Geometry: final body of the model. Coordinates: model frame, mm. Round coordinates to 2 decimals unless told otherwise and drop trailing zeros. Loops run counter-clockwise (first coordinate to the right, second up) from the corner with the lowest first, then second, coordinate; pieces in that order, holes last. Notation, with made-up numbers: (-17.5, -19) - (29.5, -19) arc R7 cw to (29.5, -12) - close; hole circle Ø5 at (84.5, -4.5). An arc over 180 degrees is marked (long way). Answer in a Markdown table with one row per item. Add a question column.
from build123d import *

# Parameters (mm, degrees)
F1_DEPTH = 37.5


with BuildPart() as f1:
    # F0 (on Top) → F1 (new body, symmetric)
    with BuildSketch(Plane.XY):
        with BuildLine():
            Line((31.333245, 3.038192), (31.333245, 17.012404))
            ThreePointArc((31.333245, 17.012404), (27.477213, 16.783619), (23.63672, 16.368966))
            Line((23.63672, 16.368966), (27.400446, 9.85))
            Line((27.400446, 9.85), (26.101409, 9.1))
            Line((26.101409, 9.1), (18.999999, 5))
            Line((18.999999, 5), (17.700962, 4.25))
            Line((17.700962, 4.25), (12.093028, 13.963227))
            ThreePointArc((12.093028, 13.963227), (-12.287424, 2.210049), (-31.35356, -17.000001))
            Line((-31.35356, -17.000001), (-1.332891, -17.000001))
            ThreePointArc((-1.332891, -17.000001), (12.760499, -3.329794), (31.333245, 3.038192))
        make_face()
    extrude(amount=F1_DEPTH, both=True)


solid = f1.part
1) Section C-C, the plane x = -24.5. Return the cut outline in (y, z), and give its area (3 significant figures).
2) Material intervals for line 1 along X through (y, z) = (8.5, 16.5); line 2 along X through (y, z) = (9, 16); line 3 along X through (y, z) = (-1, -4), sorted ascending. Write a range as from..to.
3) Contact query for flat-ended pins moving along their axis: pin 1 Ø3 at (y, z) = (0.5, 11.5) entering from -X; pin 2 Ø12 at (x, z) = (6, 14.5) entering from -Y; pin 3 Ø5 at (x, z) = (22.5, -17.5) entering from -Y. Output: stop coordinate, or through.
4) Section B-B, the plane y = 8. Return the cut outline in (x, z).
5) Section D-D, the plane y = -10. Return the cut outline in (x, z).
6) Section A-A, the plane z = -0.5. Return the cut outline in (x, y).
7) Pull-direction query (X, two-part tool) for faces 1 (the flat face through (14.936, 9.039, 0.525)), 2 (the flat face through (0, -4, -37.5)), 3 (the cylindrical face through (27.53, 16.79, 0.52)), 4 (the flat face through (25.49, 13.16, 0.52)); classes: pulls with the +X half, pulls with the -X half, needs draft (parallel to the pull), parting line crosses it, or undercut.
Evaluation:
| question | item | result |
|---|---|---|
| 1 | outline | (-17, -37.5) - (-8.52, -37.5) - (-8.52, 37.5) - (-17, 37.5) - close |
| 1 | area | 636 mm² |
| 2 | line 1 | x = -1.87..15.25, 25.06..31.33 |
| 2 | line 2 | x = -0.86..14.96, 25.93..31.33 |
| 2 | line 3 | x = -16.49..17.07 |
| 3 | pin 1 | stops at x = -16.49 |
| 3 | pin 2 | stops at y = -15.08 |
| 3 | pin 3 | stops at y = 0.26 |
| 4 | outline | (-2.84, -37.5) - (15.54, -37.5) - (15.54, 37.5) - (-2.84, 37.5) - close; (24.2, -37.5) - (31.33, -37.5) - (31.33, 37.5) - (24.2, 37.5) - close |
| 5 | outline | (-25.84, -37.5) - (4.34, -37.5) - (4.34, 37.5) - (-25.84, 37.5) - close |
| 6 | outline | (-31.35, -17) - (-1.33, -17) arc R45 cw to (31.33, 3.04) - (31.33, 17.01) arc R80 ccw to (23.64, 16.37) - (27.4, 9.85) - (26.1, 9.1) - (19, 5) - (17.7, 4.25) - (12.09, 13.96) arc R80 ccw to start |
| 7 | face 1 | undercut |
| 7 | face 2 | needs draft |
| 7 | face 3 | pulls with the -X half |
| 7 | face 4 | undercut |
